Could you check a few things on this model? Use its own coordinates, in mm. A direction names the side the tool comes from. Coordinates: 2 decimals unless noted, no trailing zeros. Loops run counter-clockwise (first coordinate to the right, second up) from the corner with the lowest first, then second, coordinate; pieces in that order, holes last. Notation, with made-up numbers: (44, -5) - (56, -5) arc R22 cw to (56, 32) - close; hole circle Ø8 at (18.5, -30). An arc over 180 degrees is marked (long way). Use CSV: the item, a comma, the result in double quotes.
from build123d import *

# Parameters (mm, degrees)
SKETCH1_R           = 2.6162
BOSS_EXTRUDE1_DEPTH = 2.159
SKETCH2_R           = 3.429
CUT_EXTRUDE1_DEPTH  = 32.658081505
FILLET1_R           = 10.16
SKETCH3_W           = 1.016
SKETCH3_H           = 17.78
BOSS_EXTRUDE2_DEPTH = 2.032
SKETCH4_R           = 3.9878
SKETCH4_R_2         = 2.6162
BOSS_EXTRUDE3_DEPTH = 2.667
FILLET2_R           = 7.62
SKETCH6_W           = 0.381
SKETCH6_H           = 28.956
CUT_EXTRUDE2_DEPTH  = 32.950948649


with BuildPart() as part:
    # Sketch1 → Boss-Extrude1 (new body)
    with BuildSketch(Plane.XY):
        Polygon((-1.016, -8.255), (-8.9916, -8.255), (-8.9916, 26.035), (-1.016, 26.035), (9.906, 26.035), (17.8816, 26.035), (17.8816, -8.255), (9.906, -8.255), align=None)
        with Locations((13.8938, 8.89)):
            Circle(SKETCH1_R, mode=Mode.SUBTRACT)
        with Locations((-5.0038, 8.89)):
            Circle(SKETCH1_R, mode=Mode.SUBTRACT)
        Polygon((0, 0), (0, 17.78), (3.048, 17.78), (3.048, 23.368), (-1.016, 23.368), (-1.016, 18.288), (-1.016, 0.508), (-1.016, -5.588), (3.016124998, -5.588), (3.016124998, 0), align=None, mode=Mode.SUBTRACT)
        Polygon((8.89, 0), (8.89, 17.78), (5.842, 17.78), (5.842, 23.368), (9.906, 23.368), (9.906, 17.78), (9.906, 0), (9.906, -5.588), (5.842, -5.588), (5.842, 0), align=None, mode=Mode.SUBTRACT)
    extrude(amount=BOSS_EXTRUDE1_DEPTH)

    # Sketch2 → Cut-Extrude1 (cut, through all)
    with BuildSketch(Plane.XY.offset(2.159)):
        with Locations((4.445, 8.89)):
            Circle(SKETCH2_R)
    extrude(amount=-CUT_EXTRUDE1_DEPTH, mode=Mode.SUBTRACT)

    # Fillet1
    fillet1_edges = [part.edges().sort_by_distance(p)[0] for p in [
        (17.8816, -8.255, 1.0795),
        (-8.9916, -8.255, 1.0795),
        (-8.9916, 26.035, 1.0795),
        (17.8816, 26.035, 1.0795),
    ]]
    fillet(fillet1_edges, radius=FILLET1_R)

    # Sketch3 → Boss-Extrude2 (add)
    with BuildSketch(Plane.XY.offset(2.159)):
        with Locations((0.508, 8.89)):
            Rectangle(SKETCH3_W, SKETCH3_H)
        with Locations((8.382, 8.89)):
            Rectangle(SKETCH3_W, SKETCH3_H)
    extrude(amount=BOSS_EXTRUDE2_DEPTH)

    # Sketch4 → Boss-Extrude3 (add)
    # profile 1 of 2: a face of its own
    with BuildSketch(Plane.XY.offset(2.159)):
        with Locations((-5.0038, 8.89)):
            Circle(SKETCH4_R)
        with Locations((-5.0038, 8.89)):
            Circle(SKETCH4_R_2, mode=Mode.SUBTRACT)
    # profile 2 of 2: a face of its own
    with BuildSketch(Plane.XY.offset(2.159)):
        with Locations((13.8938, 8.89)):
            Circle(SKETCH4_R)
        with Locations((13.8938, 8.89)):
            Circle(SKETCH4_R_2, mode=Mode.SUBTRACT)
    extrude(amount=BOSS_EXTRUDE3_DEPTH)

    # Fillet2
    # the kernel refuses this fillet: 7.62 mm, written as the material it takes off along each edge
    with BuildSketch(Plane(origin=(8.89, 0, -15.24), x_dir=(0, 1, 0), z_dir=(0, 0, 1))) as fillet2_piece_1:
        with BuildLine():
            CenterArc((6.096, 7.62), FILLET2_R, 216.869897646, 53.130102354)
            Line((0, 3.048), (-0.12192, 2.95656))
            ThreePointArc((-0.12192, 2.95656), (-0.1524, 1.524), (-0.1524, 0))
            Line((-0.1524, 0), (0, -0.1524))
            Line((0, -0.1524), (6.096, -0.1524))
            Line((6.096, -0.1524), (6.096, 0))
        make_face()
    extrude(amount=34.671, mode=Mode.SUBTRACT)
    with BuildSketch(Plane(origin=(0, 0, -15.17990756), x_dir=(0, 1, 0), z_dir=(0, 0, 1))) as fillet2_piece_2:
        with BuildLine():
            CenterArc((6.071963024, -7.62), FILLET2_R, 90, 52.82992082)
            Line((0, -3.016124998), (-0.12143926, -2.924047498))
            ThreePointArc((-0.12143926, -2.924047498), (-0.1524, -1.508062499), (-0.1524, 0))
            Line((-0.1524, 0), (0, 0.1524))
            Line((0, 0.1524), (6.071963024, 0.1524))
            Line((6.071963024, 0.1524), (6.071963024, 0))
        make_face()
    extrude(amount=34.550815121, mode=Mode.SUBTRACT)
    with BuildSketch(Plane(origin=(0, 17.78, 19.431), x_dir=(1, 0, 0), z_dir=(0, 0, -1)), Plane(origin=(8.89, 17.78, -15.24), x_dir=(-1, 0, 0), z_dir=(0, 0, 1))) as fillet2_piece_3:
        with BuildLine():
            CenterArc((7.62, 6.096), FILLET2_R, 180, 53.130102354)
            Line((0, 6.096), (-0.1524, 6.096))
            Line((-0.1524, 6.096), (-0.1524, 0))
            Line((-0.1524, 0), (0, -0.1524))
            ThreePointArc((0, -0.1524), (1.524, -0.1524), (2.95656, -0.12192))
            Line((2.95656, -0.12192), (3.048, 0))
        make_face()
    extrude(amount=34.671, mode=Mode.SUBTRACT)

    # Sketch6 → Cut-Extrude2 (cut, through all)
    with BuildSketch(Plane(origin=(0, 0, 0), x_dir=(-1, 0, 0), z_dir=(0, 0, -1))):
        with Locations((1.2065, 8.89)):
            Rectangle(SKETCH6_W, SKETCH6_H)
        with Locations((-10.0965, 8.89)):
            Rectangle(SKETCH6_W, SKETCH6_H)
    extrude(amount=-CUT_EXTRUDE2_DEPTH, mode=Mode.SUBTRACT)


solid = part.part
(1) Suppose I cut it at A-A (z = 3.65). Write out the boundary of the cut face in (x, y).
Computed:
outline,"(-1.4, 7.19) - (-1.4, 10.59) arc R3.99 ccw (long way) to start; (0, 6.07) arc R7.62 ccw to (1.02, 2.27) - (1.02, 15.49) arc R7.62 ccw to (0, 11.68) - close; (7.87, 2.29) arc R7.62 ccw to (8.89, 6.1) - (8.89, 11.68) arc R7.62 ccw to (7.87, 15.49) - close; (10.29, 7.19) arc R3.99 ccw (long way) to (10.29, 10.59) - close; hole circle Ø5.23 at (-5, 8.89); hole circle Ø5.23 at (13.89, 8.89)"
(2) Suppose I cut it at D-D (z = 0.75). Write out the boundary of the cut face in (x, y) (3 decimals), plus the area to 3 significant figures.
Computed:
outline,"(-8.992, 1.905) arc R10.16 ccw to (1.168, -8.255) - (7.722, -8.255) arc R10.16 ccw to (17.882, 1.905) - (17.882, 15.875) arc R10.16 ccw to (7.722, 26.035) - (1.168, 26.035) arc R10.16 ccw to (-8.992, 15.875) - close; hole circle Ø5.232 at (-5.004, 8.89); hole (-1.397, -5.588) - (3.016, -5.588) - (3.016, 0) arc R7.62 cw to (0, 6.072) - (0, 11.684) arc R7.62 cw to (3.048, 17.78) - (3.048, 23.368) - (-1.397, 23.368) - close; hole circle Ø6.858 at (4.445, 8.89); hole (5.842, -5.588) - (10.287, -5.588) - (10.287, 23.368) - (5.842, 23.368) - (5.842, 17.78) arc R7.62 cw to (8.89, 11.684) - (8.89, 6.096) arc R7.62 cw to (5.842, 0) - close; hole circle Ø5.232 at (13.894, 8.89)"
area,"582 mm²"
(3) Will these pins go through, and if not, where does the flat tip stop? pin 1 (1.1 mm diameter, centred on x = 8.5, z = 1, fed in from +Y); pin 2 (1 mm diameter, centred on x = 3.5, z = 3.5, fed in from +Y); pin 3 (2 mm diameter, centred on y = 0, z = 2, fed in from +X); pin 4 (8.5 mm diameter, centred on x = 5.5, y = 1, fed in from +Z).
Computed:
pin 1,"stops at y = 26.03"
pin 2,"passes through"
pin 3,"stops at x = 17.84"
pin 4,"stops at z = 4.19"
(4) Suppose I cut it at B-B (x = 4.5). Write out the boundary of the cut face in (y, z) (3 decimals).
Computed:
outline,"(-8.255, 0) - (5.461, 0) - (5.461, 2.159) - (-8.255, 2.159) - close; (12.319, 0) - (26.035, 0) - (26.035, 2.159) - (12.319, 2.159) - close"
(5) Suppose I cut it at C-C (y = 3.5). Write out the boundary of the cut face in (x, z), plus the area to 3 significant figures.
Computed:
outline,"(-8.99, 0) - (-1.4, 0) - (-1.4, 2.16) - (-8.99, 2.16) - close; (0.45, 0) - (8.43, 0) - (8.43, 4.19) - (7.87, 4.19) - (7.87, 2.16) - (1.02, 2.16) - (1.02, 4.19) - (0.45, 4.19) - close; (10.29, 0) - (17.88, 0) - (17.88, 2.16) - (10.29, 2.16) - close"
area,"52.3 mm²"
(6) Please list where these lines run through material, in increasing order: line 1 (X direction, y = 21.5, z = 1.7); line 2 (Y direction, x = 7, z = 1.7) (3 decimals); line 3 (X direction, y = -5, z = 0.2).
Computed:
line 1,"x = -7.29 to -1.4, 3.05 to 5.84, 10.29 to 16.18"
line 2,"y = -8.255 to -5.588, 1.073 to 6.603, 11.177 to 16.707, 23.368 to 26.035"
line 3,"x = -6.28 to -1.4, 3.02 to 5.84, 10.29 to 15.17"
(7) Which directions (+Z, -Z, +X, -X, +Y, -Y) give clear straight access to the entire face, cutting with the end or side of a thin tool? Please do faces 1 (the face through (-1.397, 9, 1)), 2 (the face through (1.016, 9, 3)), 3 (the face through (-8.99, 9.04, 3.47)), 4 (the face through (-7, 11, 4.826)).
Computed:
face 1,"+Z, -Z"
face 2,"+Z, +Y, -Y"
face 3,"+Z"
face 4,"+Z, +X, -X, +Y, -Y"
(8) Thinking about a two-plate mould opening in X: for faces 5 (the face through (17.882, 9, 1)), 6 (the face through (17.88, 8.74, 3.47)), 7 (the face through (17, 9, 4.826)), 8 (the face through (-6.094, 22.98, 1.095)), which applies, +X half, -X half, draft (parallel to the pull), parting line (faces both ways), or undercut?
Computed:
face 5,"+X half"
face 6,"undercut"
face 7,"draft"
face 8,"-X half"
